Here's the drawing with two shaded views (mm, measured from the low corner). I have some questions. A direction names the side the tool comes from. Give positions to 0.01 mm unless a question says otherwise; leave off trailing zeros. Loops run counter-clockwise (first coordinate to the right, second up) from the corner with the lowest first, then second, coordinate; pieces in that order, holes last. Notation, with made-up numbers: (-27, 75.25) - (-6, 75.25) arc R15 cw to (-6, 93.25) - close; hole circle Ø10 at (-28, 54). An arc over 180 degrees is marked (long way). Answer as a JSON object with one key per item and string values. Group by question number.
Item 1: Which directions (+Z, -Z, +X, -X, +Y, -Y) give clear straight access to the entire face, cutting with the end or side of a thin tool? Please do the marked faces 1, 2 and 3.
Item 2: Suppose I cut it at A-A on x = 50.8. Write out the boundary of the cut face in (y, z).
Item 3: Suppose I cut it at B-B on z = 50.8. Write out the boundary of the cut face in (x, y).
Item 4: Please list where these lines run through material, in increasing order: L1, parallel to Y at x = 17.5, z = 88; L2, parallel to Z at x = 64, y = 55.5; L3, parallel to Z at x = 55, y = 18.5.
Item 5: Suppose I cut it at C-C on y = 10. Write out the boundary of the cut face in (x, z), and give its area (3 significant figures).
Item 6: Will these pins go through, and if not, where does the flat tip stop? pin 1 (1.5 mm diameter, centred on y = 50.5, z = 62.5, fed in from +X); pin 2 (8 mm diameter, centred on x = 27, z = 28.5, fed in from -Y); pin 3 (2 mm diameter, centred on y = 10.5, z = 34, fed in from -X); pin 4 (3 mm diameter, centred on y = 33, z = 47.5, fed in from -X).
Item 7: Suppose I cut it at D-D on y = 53.5. Write out the boundary of the cut face in (x, z).
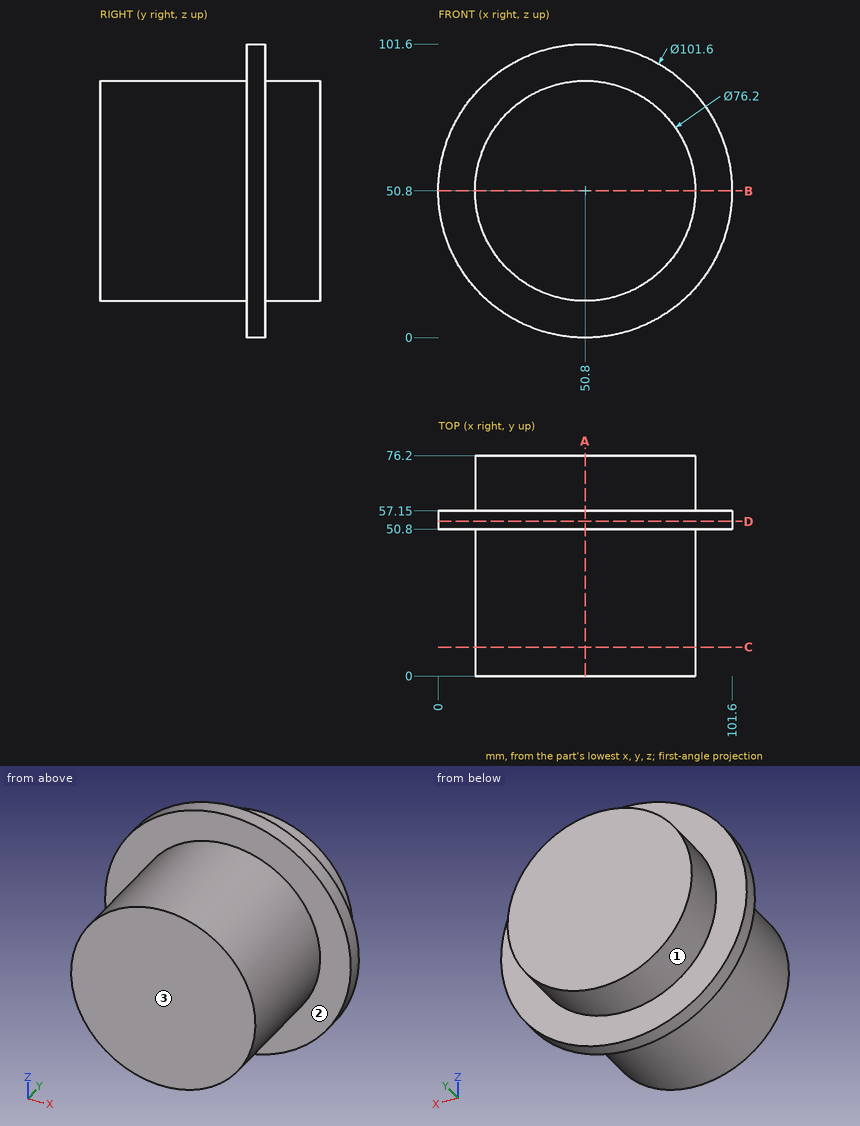
Worked out:
{
 "1": {"face 1": "+Y", "face 2": "-Y", "face 3": "+Z, -Z, +X, -X, -Y"},
 "2": {"outline": "(0, 12.7) - (50.8, 12.7) - (50.8, 0) - (57.15, 0) - (57.15, 12.7) - (76.2, 12.7) - (76.2, 88.9) - (57.15, 88.9) - (57.15, 101.6) - (50.8, 101.6) - (50.8, 88.9) - (0, 88.9) - close"},
 "3": {"outline": "(0, 50.8) - (12.7, 50.8) - (12.7, 0) - (88.9, 0) - (88.9, 50.8) - (101.6, 50.8) - (101.6, 57.15) - (88.9, 57.15) - (88.9, 76.2) - (12.7, 76.2) - (12.7, 57.15) - (0, 57.15) - close"},
 "4": {"L1": "y = 50.8 to 57.15", "L2": "z = 1.74 to 99.86", "L3": "z = 12.93 to 88.67"},
 "5": {"outline": "circle Ø76.2 at (50.8, 50.8)", "area": "4,560 mm2"},
 "6": {"pin 1": "stops at x = 100.39", "pin 2": "stops at y = 0", "pin 3": "stops at x = 16.13", "pin 4": "stops at x = 12.74"},
 "7": {"outline": "circle Ø101.6 at (50.8, 50.8)"}
}
